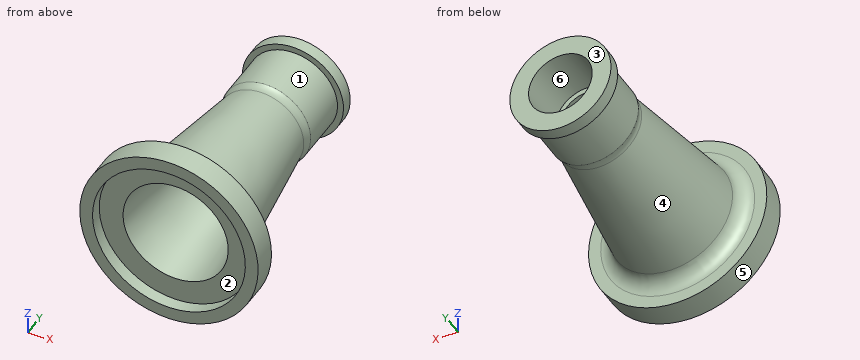
```python
from build123d import *

# Parameters (mm, degrees)
FILLET1_R = 12
FILLET2_R = 12


with BuildPart() as part:
    # Sketch2 → Revolve-Thin2 (revolve)
    with BuildSketch(Plane.XY, mode=Mode.PRIVATE) as revolve_thin2_sk:
        Polygon((39.725895331, 131.026369151), (35, 131.026369151), (35, 91.026369151), (32.5, 91.026369151), (50, -33.973630849), (70, -33.973630849), (70, -53.973630849), (60, -53.973630849), (60, -43.973630849), (41.302475551, -43.973630849), (21.002475551, 101.026369151), (25, 101.026369151), (25, 141.026369151), (39.725895331, 141.026369151), align=None)
    revolve(revolve_thin2_sk.sketch.rotate(Axis((0, -92.5, 0), (0, 1, 0)), 90), axis=Axis((0, -92.5, 0), (0, 1, 0)))

    # Fillet1
    # the kernel refuses this fillet: 12 mm, written as the material it adds along each edge
    with BuildSketch(Plane(origin=(0, 91.026369151, 0), x_dir=(0, 0, -1), z_dir=(1, 0, 0))) as fillet1_piece_1:
        with BuildLine():
            CenterArc((45.444294459, -5.909036575), FILLET1_R, 150.500253151, 37.469357243)
            Line((33.560193499, -7.572810709), (33.32251148, -7.606086192))
            Line((33.32251148, -7.606086192), (32.262317981, -0.033275483))
            Line((32.262317981, -0.033275483), (32.5, 0.24))
            ThreePointArc((32.5, 0.24), (33.75, 0.24), (34.791114111, 0.118180731))
            Line((34.791114111, 0.118180731), (35, 0))
        make_face()
    revolve(axis=Axis((0, 91.026369151, 0), (0, 1, 0)))

    # Fillet2
    fillet2_edges = [part.edges().sort_by_distance(p)[0] for p in [
        (0, -33.973630849, 50),
    ]]
    fillet(fillet2_edges, radius=FILLET2_R)


solid = part.part
```
Read the model definition and answer for the solid it produces. Units are mm, in the model's axes. Face numbers are marked on the shaded views. A direction names the side the tool comes from. Give positions to 0.01 mm unless a question says otherwise; leave off trailing zeros. Loops run counter-clockwise (first coordinate to the right, second up) from the corner with the lowest first, then second, coordinate; pieces in that order, holes last.
Item 1: The part is cut by section C-C (y = 128). Write down the section's boundary in (x, z), and give its area (3 significant figures).
Item 2: Each of these flat-tipped pins is pushed along its axis until it touches: pin 1 Ø10 at (y, z) = (63.5, -8) entering from +X; pin 2 Ø1 at (y, z) = (-4.5, 5.5) entering from +X. Where does it stop, or does it pass through?
Item 3: The part is cut by section D-D (y = -37). Write down the section's boundary in (x, z), and give its area (3 significant figures).
Item 4: Find the intervals of material crossed by line 1 along X through (y, z) = (123, 0); line 2 along X through (y, z) = (132, 0); line 3 along Z through (x, y) = (0.5, 48.5), in increasing order.
Item 5: The mould has two halves that part along X. Classify the marked faces 1, 2 and 3: released by +X, released by -X, zero draft, split by the parting line, or undercut.
Item 6: For the marked faces 4, 5 and 6, determine the directions among +Z, -Z, +X, -X, +Y, -Y from which every point of the face is accessible in a straight line to the end or side of a thin tool.
Taken from the geometry:
1. outline: circle Ø70 at (0, 0); hole circle Ø50 at (0, 0)
1. area: 1,880 mm2
2. pin 1: stops at x = 36.58
2. pin 2: stops at x = 45.63
3. outline: circle Ø140 at (0, 0); hole circle Ø80.65 at (0, 0)
3. area: 10,300 mm2
4. line 1: x = -35 to -25, 25 to 35
4. line 2: x = -39.73 to -25, 25 to 39.73
4. line 3: z = -38.45 to -28.35, 28.35 to 38.45
5. face 1: split by the parting line
5. face 2: undercut
5. face 3: zero draft
6. face 4: none
6. face 5: +Y, -Y
6. face 6: +Y
